Could you check a few things on this drawing? It's one solid part, dimensions in mm from its lowest x, y, z. A direction names the side the tool comes from. Round coordinates to 2 decimals unless told otherwise and drop trailing zeros. Write each loop counter-clockwise with the first axis right and the second up, starting at its lowest first coordinate (ties: lowest second). Pieces come first, ordered by that corner, then holes. Notation, with made-up numbers: (60.25, 89.25) -> (108.25, 89.25) arc R14 ccw to (108.25, 102.25) -> close; hole circle Ø5 at (61, 37.5). An arc over 180 degrees is marked (long way). Answer in a Markdown table with one row per item.
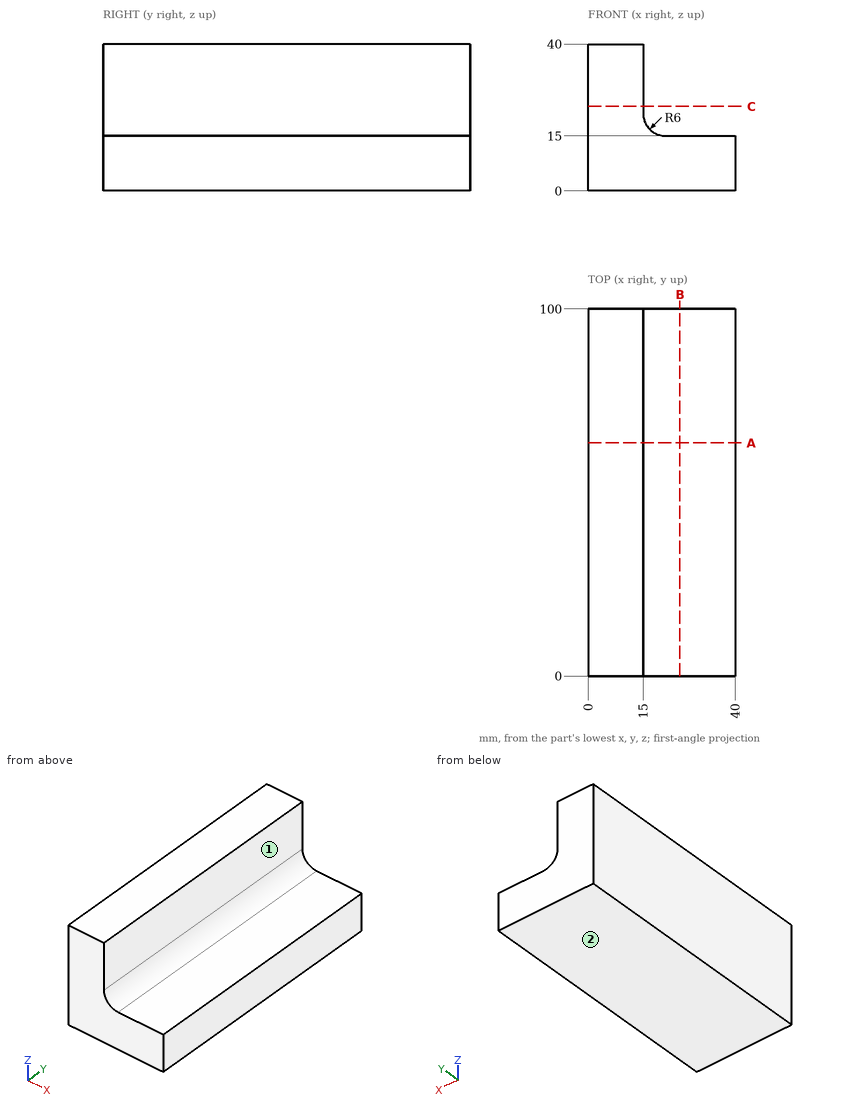
1) I want a section at C-C, the plane z = 23. List the corners of the cut face in (x, y) for me.
Response:
| item | result |
|---|---|
| outline | (0, 0) -> (15, 0) -> (15, 100) -> (0, 100) -> close |
2) I need wall thicknesses on line 1 (Z direction, x = 25, y = 18); line 2 (Z direction, x = 16.5, y = 40). Which ranges of each line are inside material? Lowest first, please. Write a range as [from, to].
Response:
| item | result |
|---|---|
| line 1 | z = [0, 15] |
| line 2 | z = [0, 17.03] |
3) For pin 1 (3 mm diameter, centred on x = 36, y = 62.5, fed in from +Z); pin 2 (21 mm diameter, centred on y = 40, z = 29.5, fed in from +X); pin 3 (6 mm diameter, centred on y = 36, z = 36, fed in from +X); pin 4 (2 mm diameter, centred on y = 39.5, z = 32.5, fed in from -X), each with a flat end and sliding along its axis, tell me the tip position at first contact or that it passes through.
Response:
| item | result |
|---|---|
| pin 1 | stops at z = 15 |
| pin 2 | stops at x = 15.34 |
| pin 3 | stops at x = 15 |
| pin 4 | stops at x = 0 |
4) I want a section at B-B, the plane x = 25. List the corners of the cut face in (y, z) for me, and give its area (3 significant figures).
Response:
| item | result |
|---|---|
| outline | (0, 0) -> (100, 0) -> (100, 15) -> (0, 15) -> close |
| area | 1,500 mm^2 |
5) Which directions (+Z, -Z, +X, -X, +Y, -Y) give clear straight access to the entire face, cutting with the end or side of a thin tool? Please do the marked faces 1 and 2.
Response:
| item | result |
|---|---|
| face 1 | +Z, +X, +Y, -Y |
| face 2 | -Z, +X, -X, +Y, -Y |
6) I want a section at A-A, the plane y = 63.5. List the corners of the cut face in (x, z) for me, and give its area (3 significant figures).
Response:
| item | result |
|---|---|
| outline | (0, 0) -> (40, 0) -> (40, 15) -> (21, 15) arc R6 cw to (15, 21) -> (15, 40) -> (0, 40) -> close |
| area | 983 mm^2 |
